For this review, take the finished solid that the model builds, in its own axes (mm). A direction names the side the tool comes from. Give positions to 0.01 mm unless a question says otherwise; leave off trailing zeros. Write each loop counter-clockwise with the first axis right and the second up, starting at its lowest first coordinate (ties: lowest second). Pieces come first, ordered by that corner, then holes.
1) Draft analysis for pull direction Z (two halves, no side actions). For faces 4 (the face through (2.86, -31.89, -21.74)), 5 (the face through (1.268, 21.088, 19.614)), 6 (the face through (1, 50, 19)), state which applies: pulls with the +Z half, pulls with the -Z half, needs draft (parallel to the pull), parting line crosses it, or undercut.
2) We need section C-C on x = 0.9. Give the number of separate pieces and of enclosed holes in the cut face, and give its area (3 significant figures).
3) For P1, Ø3.5, axis at y = 45, z = -20, coming from the +X side; P2, Ø1.5, axis at x = 2.5, z = -1, coming from the +Y side; P3, Ø6, axis at y = 8, z = -11, coming from the -X side; P4, Ø4, axis at y = 45, z = 20, coming from the -X side, all flat-tipped, find the tip position at first contact; note any pin that passes through.
4) Machinability: for faces 1 (the face through (1, 12, 25)), 2 (the face through (2.635, 21.351, -19.802)), 3 (the face through (1.27, 21.38, -19.67)), which of the approach directions +Z, -Z, +X, -X, +Y, -Y give a long, thin tool a straight path to every point of the face, cutting with its end or side? Answer none if there is none.
5) Wall thickness on line 1 along Z through (x, y) = (2.3, 44); line 2 along Z through (x, y) = (2.8, -26.5) (3 decimals); line 3 along Z through (x, y) = (0.25, 24.5): over which ranges is each line inside the solid? List them lowest first.
6) We need section D-D on y = 45. Give the boundary of the cut face in (x, z), and give its area (3 significant figures).
7) We need section A-A on y = -10. Give the boundary of the cut face in (x, z).
8) We need section B-B on z = 0. Give the boundary of the cut face in (x, y), and give its area (3 significant figures).
from build123d import *

# Parameters (mm, degrees)
SKETCH_1_W          = 50
SKETCH_1_H          = 85
EXTRUDE_1_DEPTH     = 3
FILLET_2_R          = 10
SKETCH_4_R          = 1.5
CUT_EXTRUDE_1_DEPTH = 3
CHAMFER_1_SIZE      = 0.5
CUT_EXTRUDE_3_DEPTH = 3
SKETCH_7_R          = 22.5
CUT_EXTRUDE_4_DEPTH = 3
FILLET_4_R          = 4
CHAMFER_2_SIZE      = 0.5
CHAMFER_3_SIZE      = 0.5


with BuildPart() as part:
    # 草图1 → 凸台-拉伸1 (new body)
    with BuildSketch(Plane(origin=(0, 0, 0), x_dir=(0, 0, -1), z_dir=(1, 0, 0))):
        with Locations((0, 7.5)):
            Rectangle(SKETCH_1_W, SKETCH_1_H)
    extrude(amount=EXTRUDE_1_DEPTH)

    # 圆角2
    fillet_2_edges = [part.edges().sort_by_distance(p)[0] for p in [
        (1.5, -35, -25),
        (1.5, -35, 25),
    ]]
    fillet(fillet_2_edges, radius=FILLET_2_R)

    # 草图4 → 切除-拉伸1 (cut)
    with BuildSketch(Plane(origin=(3, 0, 0), x_dir=(0, 0, -1), z_dir=(1, 0, 0))):
        with Locations((20, 45)):
            Circle(SKETCH_4_R)
        with Locations((-20, 45)):
            Circle(SKETCH_4_R)
        with Locations((-18, -28)):
            Circle(SKETCH_4_R)
    extrude(amount=-CUT_EXTRUDE_1_DEPTH, mode=Mode.SUBTRACT)

    # 倒角1
    chamfer_1_edges = [part.edges().sort_by_distance(p)[0] for p in [
        (3, 12.5, -25),
        (3, 50, 0),
        (3, -35, 0),
        (3, -32.071067812, 22.071067812),
        (3, -32.071067812, -22.071067812),
        (3, 12.5, 25),
    ]]
    chamfer(chamfer_1_edges, length=CHAMFER_1_SIZE)

    # 草图6 → 切除-拉伸3 (cut)
    with BuildSketch(Plane(origin=(3, 0, 0), x_dir=(0, 0, -1), z_dir=(1, 0, 0))):
        with BuildLine():
            Line((-12.5, 50), (12.5, 50))
            Line((12.5, 50), (18.896399481, 31.551800259))
            ThreePointArc((18.896399481, 31.551800259), (0, 5), (-18.896399481, 31.551800259))
            Line((-18.896399481, 31.551800259), (-12.5, 50))
        make_face()
    extrude(amount=-CUT_EXTRUDE_3_DEPTH, mode=Mode.SUBTRACT)

    # 草图7 → 切除-拉伸4 (cut)
    with BuildSketch(Plane(origin=(3, 0, 0), x_dir=(0, 0, -1), z_dir=(1, 0, 0))):
        with Locations((0, -10)):
            Circle(SKETCH_7_R)
    extrude(amount=-CUT_EXTRUDE_4_DEPTH, mode=Mode.SUBTRACT)

    # 圆角4
    fillet_4_edges = [part.edges().sort_by_distance(p)[0] for p in [
        (1.5, 9.017857143, 12.02377269),
        (1.5, 9.017857143, -12.02377269),
    ]]
    fillet(fillet_4_edges, radius=FILLET_4_R)

    # 倒角2
    chamfer_2_edges = [part.edges().sort_by_distance(p)[0] for p in [
        (3, 45, -18.5),
        (3, 45, 21.5),
        (3, -28, 19.5),
    ]]
    chamfer(chamfer_2_edges, length=CHAMFER_2_SIZE)

    # 倒角3
    chamfer_3_edges = [part.edges().sort_by_distance(p)[0] for p in [
        (3, 40.52590013, -15.784880278),
        (3, 21.231347471, -19.641722382),
        (3, 9.097355452, -14.160817784),
        (3, -32.5, 0),
        (3, 40.52590013, 15.784880278),
        (3, 9.097355452, 14.160817784),
        (3, 21.231347471, 19.641722382),
    ]]
    chamfer(chamfer_3_edges, length=CHAMFER_3_SIZE)


solid = part.part
Results list:
1. face 4: pulls with the -Z half
1. face 5: undercut
1. face 6: needs draft
2. separate pieces: 1
2. enclosed holes: 3
2. area: 1,240 mm2
3. P1: stops at x = 2.75
3. P2: stops at y = -32.43
3. P3: passes through
3. P4: stops at x = 0
4. face 1: +Z, +X, -X, +Y, -Y
4. face 2: +X
4. face 3: +X, -X
5. line 1: z = -25 to -21.12, -18.88 to -14.58, 14.58 to 18.88, 21.12 to 25
5. line 2: z = -24.583 to -15.735, 15.735 to 17.005, 18.995 to 24.583
5. line 3: z = -25 to -19.99, 19.99 to 25
6. outline: (0, -25) - (2.5, -25) - (3, -24.5) - (3, -22) - (2.5, -21.5) - (0, -21.5) - close; (0, -18.5) - (2.5, -18.5) - (3, -18) - (3, -14.76) - (2.5, -14.23) - (0, -14.23) - close; (0, 14.23) - (2.5, 14.23) - (3, 14.76) - (3, 18) - (2.5, 18.5) - (0, 18.5) - close; (0, 21.5) - (2.5, 21.5) - (3, 22) - (3, 24.5) - (2.5, 25) - (0, 25) - close
6. area: 45.6 mm2
7. outline: (0, -25) - (2.5, -25) - (3, -24.5) - (3, -23) - (2.5, -22.5) - (0, -22.5) - close; (0, 22.5) - (2.5, 22.5) - (3, 23) - (3, 24.5) - (2.5, 25) - (0, 25) - close
8. outline: (0, -35) - (2.5, -35) - (3, -34.5) - (3, -33) - (2.5, -32.5) - (0, -32.5) - close
8. area: 7.25 mm2
